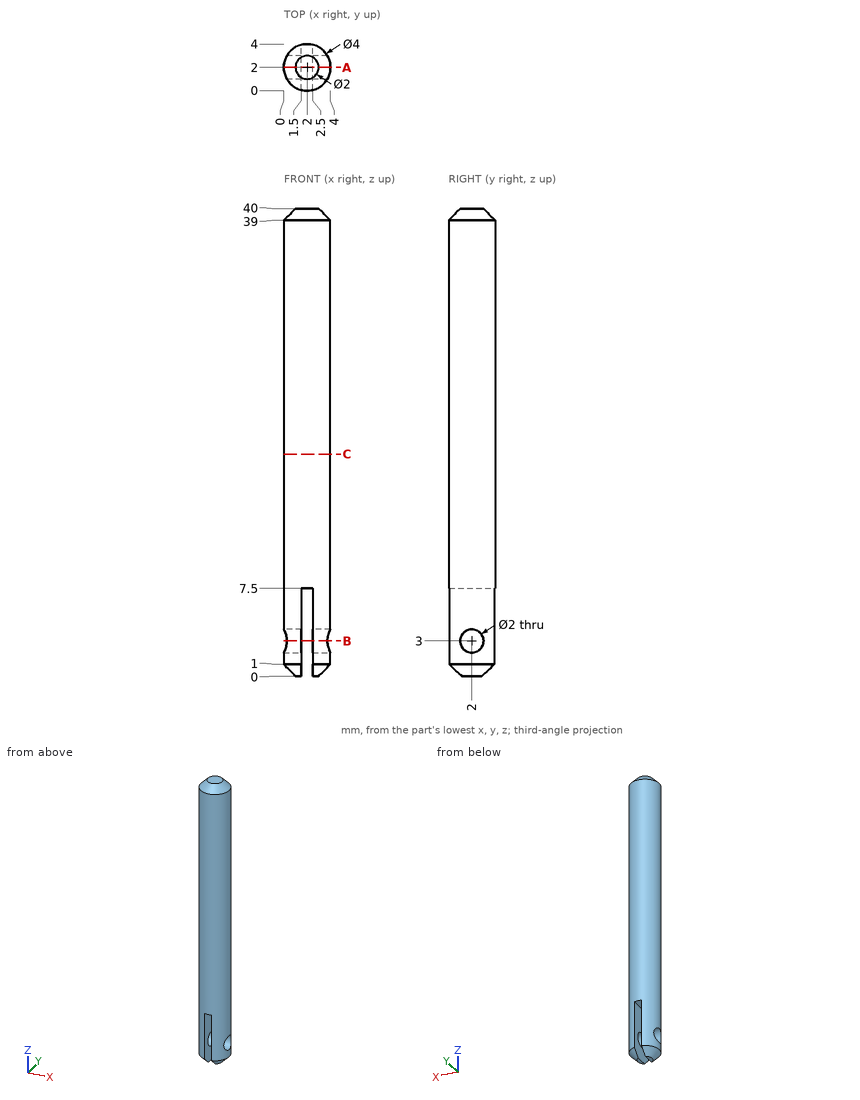
Geometry check sheet. Reference: drawing and pictorial views, mm from the part's lowest x, y, z. Coordinates: 2 decimals unless noted, no trailing zeros. Loops run counter-clockwise (first coordinate to the right, second up) from the corner with the lowest first, then second, coordinate; pieces in that order, holes last.
1) Material ranges on probe 1 along Z at (x, y) = (2.45, 1.65); probe 2 along Y at (x, z) = (3.05, 3); probe 3 along Y at (x, z) = (0.2, 37), recorded low to high.
2) Sectioned sample at B-B (z = 3). Record the boundary of the cut face in (x, y).
3) Gauge pin test, flat end, axial feed: pin 1 (0.8 mm diameter, centred on x = 2, y = 1.5, fed in from -Z). Record the tip position at first contact, or that the pin passes through.
4) Sectioned sample at A-A (y = 2). Record the boundary of the cut face in (x, z), and give its area (4 significant figures).
5) Sectioned sample at C-C (z = 19). Record the boundary of the cut face in (x, y).
Check sheet entries:
1. probe 1: z = 7.5 to 40
1. probe 2: y = 0.3 to 1, 3 to 3.7
1. probe 3: y = 1.13 to 2.87
2. outline: (0.27, 1) arc R2 ccw to (1.5, 0.06) - (1.5, 1) - close; (0.27, 3) - (1.5, 3) - (1.5, 3.94) arc R2 ccw to start; (2.5, 0.06) arc R2 ccw to (3.73, 1) - (2.5, 1) - close; (2.5, 3) - (3.73, 3) arc R2 ccw to (2.5, 3.94) - close
3. pin 1: stops at z = 7.5
4. outline: (0, 1) - (1, 0) - (1.5, 0) - (1.5, 2) - (0, 2) - close; (0, 4) - (1.5, 4) - (1.5, 7.5) - (2.5, 7.5) - (2.5, 4) - (4, 4) - (4, 39) - (3, 40) - (1, 40) - (0, 39) - close; (2.5, 0) - (3, 0) - (4, 1) - (4, 2) - (2.5, 2) - close
4. area: 144.5 mm2
5. outline: circle Ø4 at (2, 2)
